Autodesk Inventor part; units mm, degrees
ref_plane "Work Plane1" through (0, 0, -15) normal (0, 0, 1) x (1, 0, 0)
ref_plane "YZ Plane" through (0, 0, 0) normal (1, 0, 0) x (0, 1, 0)
ref_plane "XZ Plane" through (0, 0, 0) normal (0, 1, 0) x (-1, 0, 0)
sketch "Sketch1" plane through (0, 0, 0) normal (0, 0, 1) x (1, 0, 0)
  line L0 (0, 0) -> (25, 0)
  line L1 (25, 0) -> (25, 40)
  line L2 (25, 40) -> (0, 40)
  line L3 (0, 40) -> (0, 0)
  dimension "d1" = 25
  dimension "d2" = 40
  dimension "d3" = 25
extrude "Extrusion1" add sketch "Sketch1" against normal blind 30
sketch "Sketch2" plane through (25, 0, 0) normal (1, 0, 0) x (0, 0, -1)
  line L0 (0, 0) -> (30, 0)
  circle A0 centre (15, 6.56) radius 2.46
extrude "Extrusion2" cut sketch "Sketch2" against normal blind 30
sketch "Sketch3" plane through (0, 0, 0) normal (-1, 0, 0) x (0, 0, 1)
  line L0 (0, 0) -> (-30, 0)
  line L1 (-25.05, 0) -> (-4.95, 0)
  line L2 (-4.95, 0) -> (-4.95, 33.12)
  line L3 (-4.95, 33.12) -> (-25.05, 33.12)
  line L4 (-25.05, 33.12) -> (-25.05, 0)
  dimension "d11" = 20.1
extrude "Extrusion3" cut sketch "Sketch3" against normal blind 20
sketch "Sketch4" plane through (0, 0, 0) normal (0, -1, 0) x (1, 0, 0)
  line L0 (20, -4.95) -> (20, -25.05)
  line L1 (20, -15) -> (25, -15)
  line L2 (25, 0) -> (25, -30)
  line L3 (20, -8.025) -> (25, -8.025)
  line L4 (25, -8.025) -> (25, -21.975)
  line L5 (25, -21.975) -> (20, -21.975)
  line L6 (20, -21.975) -> (20, -8.025)
  line L7 (20, -8.025) -> (25, -21.975) construction
  line L8 (25, -8.025) -> (20, -21.975) construction
  line L9 (25, -12.54) -> (25, -17.46)
  point P0 (0, 0)
  point P1 (22.5, -15)
  dimension "d14" = 13.95
extrude "Extrusion4" add sketch "Sketch4" along normal blind 15
sketch "Sketch5" plane through (20, 0, 0) normal (-1, 0, 0) x (0, 0, 1)
  circle A0 centre (-15, 6.56) radius 2.46
  circle A1 centre (-15, 6.56) radius 4.7025
  circle A2 centre (-15, 6.56) radius 2.46
  circle A3 centre (-15, 6.56) radius 2.46
  point P0 (0, 0)
  dimension "d17" = 9.405
extrude "Extrusion5" cut sketch "Sketch5" against normal blind 2.1
sketch "Sketch6" plane through (25, 0, 0) normal (1, 0, 0) x (0, 0, -1)
  circle A0 centre (15, 6.56) radius 4.7025
  line L0 (15, 6.56) -> (15, 23.56)
  circle A1 centre (15, 23.56) radius 2.46
  point P0 (0, 0)
  dimension "d20" = 17
  dimension "d21" = 4.92
extrude "Extrusion6" cut sketch "Sketch6" against normal blind 10 contours A1
sketch "Sketch7" plane through (20, 0, 0) normal (-1, 0, 0) x (0, 0, 1)
  circle A0 centre (-15, 23.56) radius 2.46
  circle A1 centre (-15, 23.56) radius 4.7025
  point P0 (0, 0)
  dimension "d24" = 9.405
extrude "Extrusion7" cut sketch "Sketch7" against normal blind 2.1
sketch "Sketch9" plane through (25, 0, 0) normal (1, 0, 0) x (0, 0, -1)
  circle A0 centre (15, 6.56) radius 2.46
  circle A1 centre (15, 6.56) radius 2.46
  circle A2 centre (15, 23.56) radius 2.46
  circle A3 centre (15, 23.56) radius 2.46
  line L0 (30, 40) -> (30, 0)
  line L1 (30, 0) -> (30, 40)
  line L2 (30, 40) -> (0, 40)
  line L3 (0, 40) -> (0, 0)
  line L4 (0, 0) -> (8.025, 0)
  line L5 (21.975, 0) -> (21.975, -15)
  line L6 (21.975, -15) -> (8.025, -15)
  line L7 (8.025, -15) -> (8.025, 0)
  line L8 (0, 0) -> (8.025, 0)
  line L9 (21.975, 0) -> (30, 0)
extrude "Extrusion8" add sketch "Sketch9" along normal blind 5
sketch "Sketch10" plane through (0, 40, 0) normal (0, 1, 0) x (1, 0, 0)
  line L0 (0, 30) -> (30, 30)
  line L1 (30, 0) -> (0, 0)
  line L2 (0, 30) -> (30, 30)
  line L3 (30, 30) -> (30, 0)
  line L4 (30, 0) -> (0, 0)
  line L5 (0, 0) -> (0, 30)
extrude "Extrusion9" add sketch "Sketch10" along normal blind 30
sketch "Sketch12" plane through (30, 0, 0) normal (1, 0, 0) x (0, 0, -1)
  circle A0 centre (15, 6.56) radius 2.46
  line L0 (15, 6.56) -> (15, 15.06)
  circle A1 centre (15, 15.06) radius 2.525
  point P0 (0, 0)
  dimension "d31" = 8.5
  dimension "d33" = 5.05
extrude "Extrusion10" cut sketch "Sketch12" against normal blind 30 contours A1
sketch "Sketch14" plane through (0, 0, 0) normal (0, 0, 1) x (1, 0, 0)
  line L0 (30, 70) -> (0, 70)
  line L1 (0, 100) -> (-8, 100)
  line L2 (30, 0) -> (30, 70)
  line L3 (30, 118) -> (30, 70)
  line L4 (30, 105) -> (30, 100)
  line L5 (0, 70) -> (30, 70)
  line L6 (0, 70) -> (0, 100)
  line L7 (30, 122.5) -> (30, 118)
  line L8 (-2, 150) -> (-8, 152)
  line L9 (-2, 102) -> (-8, 100)
  line L10 (-2, 102) -> (4, 126)
  line L11 (4, 126) -> (-2, 150)
  line L12 (-8, 152) -> (15, 152)
  line L13 (30, 137) -> (15, 152)
  line L14 (30, 122.5) -> (30, 137)
  point P0 (0, 0)
  dimension "d47" = 30
extrude "Extrusion12" add sketch "Sketch14" against normal blind 30
sketch "Sketch15" plane through (0, 0, -25.05) normal (-1, 0, 0) x (0, 0, 1)
  line L0 (0, 33.12) -> (20.1, 33.12)
  line L1 (20.1, 33.12) -> (20.1, 0)
  line L2 (0, 33.12) -> (20.1, 33.12)
  line L3 (20.1, 33.12) -> (20.1, 31.1)
  line L4 (20.1, 31.1) -> (0, 31.1)
  line L5 (0, 31.1) -> (0, 33.12)
  point P0 (25.05, 0)
  dimension "d57" = 2.02
extrude "Extrusion13" add sketch "Sketch15" against normal blind 20
sketch "Sketch25" plane through (0, 0, 0) normal (0, 0, 1) x (1, 0, 0)
  point P0 (0, 0)
sketch "Sketch26" plane through (0, 0, 0) normal (0, 0, 1) x (1, 0, 0)
  line L0 (-8, 100) -> (0, 100)
  line L1 (0, 100) -> (-8, 100)
  line L2 (-8, 100) -> (-2, 102)
  line L3 (-8, 100) -> (-2, 102)
  line L4 (-2, 102) -> (4, 126)
  line L5 (-2, 102) -> (4, 126)
  line L6 (4, 126) -> (-2, 150)
  line L7 (4, 126) -> (-2, 150)
  line L8 (-8, 152) -> (-2, 150)
  line L9 (-2, 150) -> (-8, 152)
  line L10 (15, 152) -> (-8, 152)
  line L11 (-8, 152) -> (15, 152)
  line L12 (30, 137) -> (15, 152)
  line L13 (15, 152) -> (30, 137)
  line L14 (30, 137) -> (30, 92)
  line L15 (30, 0) -> (30, 137)
  line L16 (30, 92) -> (0, 92)
  line L17 (0, 0) -> (0, 100)
  line L18 (0, 100) -> (0, 92)
  dimension "d93" = 45
extrude "Extrusion14" add sketch "Sketch26" along normal blind 30
ref_plane "Work Plane1" through (0, 0, -15) normal (0, 0, 1) x (1, 0, 0)
mirror "Mirror1" about plane through (0, 0, -15) normal (0, 0, 1) of "Extrusion14"
properties part number "48mm_x_90mm"
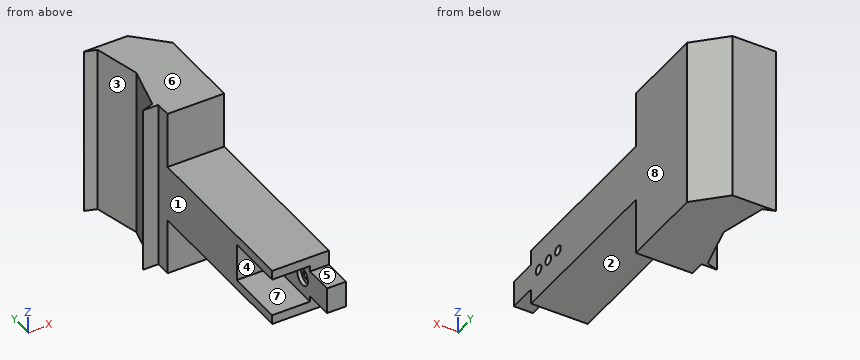
Geometry check sheet. Reference: the model listing, model coordinates, mm. Face numbers are marked on the shaded views. A direction names the side the tool comes from. Give positions to 0.01 mm unless a question says otherwise; leave off trailing zeros. Order: outer loops, then holes, each group sorted by start corner. A loop starts at its lowest first (then second) coordinate and runs counter-clockwise, first axis right, second up. Notation, with made-up numbers: (85.25, 52) - (141.25, 52) arc R5 cw to (141.25, 61) - close; hole circle Ø8 at (-10, -34.5). An arc over 180 degrees is marked (long way). Answer as a JSON object with one key per item and string values.
(1) Cross-section at D-D (z = -45). Record the cut outline in (x, y), then the cut area to 3 significant figures.
Report:
{"outline": "(-8, 100) - (0, 100) - (0, 92) - (30, 92) - (30, 137) - (15, 152) - (-8, 152) - (-2, 150) - (4, 126) - (-2, 102) - close", "area": "1,660 mm^2"}
(2) Material ranges on line 1 (Z direction, x = 21, y = 23); line 2 (Z direction, x = 27.25, y = 6.56); line 3 (Y direction, x = 25.5, z = -15) (3 decimals), recorded low to high.
Report:
{"line 1": "-30 to -19.67, -10.33 to 0", "line 2": "-30 to -17.46, -12.54 to 0", "line 3": "-15 to 4.1, 9.02 to 12.535, 17.585 to 21.1, 26.02 to 141.5"}
(3) Tool access check on the marked faces 1, 2, 3, 4 and 5. Record the directions out of +Z, -Z, +X, -X, +Y, -Y that give a thin tool (end or side, any length) a straight path to the whole face; none if there is none.
Report:
{"face 1": "+Z, -Z, -X, -Y", "face 2": "-Z, +X, -X, -Y", "face 3": "+Z, -Z, -X", "face 4": "-X, -Y", "face 5": "+Z, +X, -X, -Y"}
(4) Draft check along Z on the marked faces 6, 7 and 8. Enter one of: released by +Z, released by -Z, zero draft, split by the parting line, or undercut.
Report:
{"face 6": "released by +Z", "face 7": "undercut", "face 8": "zero draft"}
(5) Depth check by flat-ended pin: pin 1 Ø9 at (x, y) = (21.5, 58) entering from -Z; pin 2 Ø1.5 at (x, z) = (17, -20) entering from -Y; pin 3 Ø11 at (x, y) = (24, -6.5) entering from +Z (3 decimals); pin 4 Ø3 at (y, z) = (6.56, -15) entering from +X. Enter the tip coordinate at first touch or a pass-through.
Report:
{"pin 1": "z = -30", "pin 2": "y = 31.1", "pin 3": "z = -8.025", "pin 4": "through"}
(6) Cross-section at A-A (y = 15.06). Record the cut outline in (x, z) (3 decimals), then the cut area to 4 significant figures.
Report:
{"outline": "(0, -30) - (30, -30) - (30, -17.525) - (20, -17.525) - (20, -25.05) - (0, -25.05) - close; (0, -4.95) - (20, -4.95) - (20, -12.475) - (30, -12.475) - (30, 0) - (0, 0) - close", "area": "447.5 mm^2"}
(7) Cross-section at C-C (x = 8). Record the cut outline in (y, z).
Report:
{"outline": "(0, -30) - (92, -30) - (92, -60) - (152, -60) - (152, 30) - (92, 30) - (92, 0) - (0, 0) - (0, -4.95) - (31.1, -4.95) - (31.1, -25.05) - (0, -25.05) - close"}
(8) Cross-section at B-B (z = -15). State how many separate pieces and enclosed holes the cut face has, then the cut area to 3 significant figures.
Report:
{"separate pieces": "4", "enclosed holes": "0", "area": "3,780 mm^2"}
